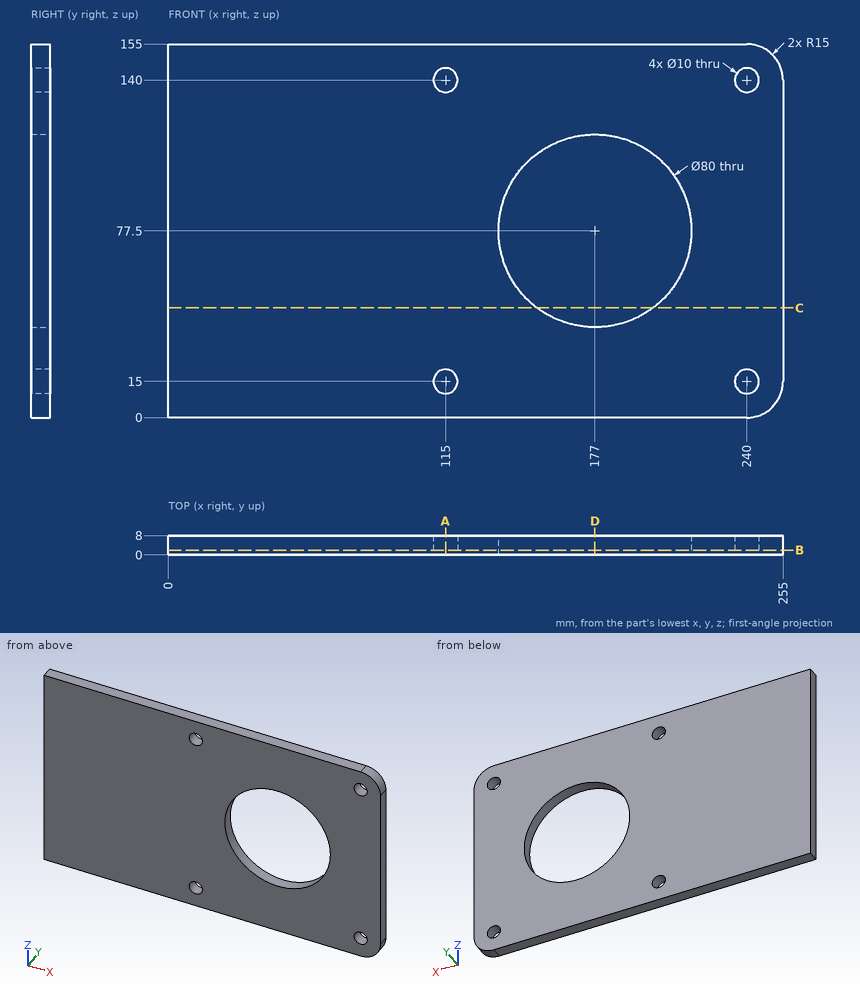
Could you check a few things on this drawing? It's one solid part, dimensions in mm from its lowest x, y, z. Round coordinates to 2 decimals unless told otherwise and drop trailing zeros. Loops run counter-clockwise (first coordinate to the right, second up) from the corner with the lowest first, then second, coordinate; pieces in that order, holes last. Notation, with made-up numbers: (-4.75, 4.5) -> (46.25, 4.5) arc R32 cw to (46.25, 38.5) -> close; hole circle Ø3 at (59, -34.5). An arc over 180 degrees is marked (long way). Answer as CSV lines item,"result".
1. If we section it at D-D on x = 177: Please give me the cut outline in (y, z), plus the area to 3 significant figures.
Final values:
outline,"(0, 0) -> (8, 0) -> (8, 37.5) -> (0, 37.5) -> close; (0, 117.5) -> (8, 117.5) -> (8, 155) -> (0, 155) -> close"
area,"600 mm^2"
2. If we section it at C-C on z = 45.5: Please give me the cut outline in (x, y).
Final values:
outline,"(0, 0) -> (153, 0) -> (153, 8) -> (0, 8) -> close; (201, 0) -> (255, 0) -> (255, 8) -> (201, 8) -> close"
3. If I drill on L1, parallel to X at y = 3.25, z = 140; L2, parallel to X at y = 2.75, z = 76.5; L3, parallel to X at y = 5, z = 135.5, over which ranges is the centre line in solid material (lowest first)?
Final values:
L1,"x = 0 to 110, 120 to 235, 245 to 255"
L2,"x = 0 to 137.01, 216.99 to 255"
L3,"x = 0 to 112.82, 117.18 to 237.82, 242.18 to 255"
4. If we section it at A-A on x = 115: Please give me the cut outline in (y, z), plus the area to 3 significant figures.
Final values:
outline,"(0, 0) -> (8, 0) -> (8, 10) -> (0, 10) -> close; (0, 20) -> (8, 20) -> (8, 135) -> (0, 135) -> close; (0, 145) -> (8, 145) -> (8, 155) -> (0, 155) -> close"
area,"1,080 mm^2"
5. For pin 1 (16 mm diameter, centred on x = 240, z = 15, fed in from -Y), with a flat end and sliding along its axis, tell me the tip position at first contact or that it passes through.
Final values:
pin 1,"stops at y = 0"
6. If we section it at B-B on y = 2: Please give me the cut outline in (x, z).
Final values:
outline,"(0, 0) -> (240, 0) arc R15 ccw to (255, 15) -> (255, 140) arc R15 ccw to (240, 155) -> (0, 155) -> close; hole circle Ø10 at (115, 15); hole circle Ø10 at (115, 140); hole circle Ø80 at (177, 77.5); hole circle Ø10 at (240, 15); hole circle Ø10 at (240, 140)"
